Geometry: final body of the model. Coordinates: model frame, mm. A direction names the side the tool comes from. Coordinates: 2 decimals unless noted, no trailing zeros. Write each loop counter-clockwise with the first axis right and the second up, starting at its lowest first coordinate (ties: lowest second). Pieces come first, ordered by that corner, then holes.
from build123d import *

# Parameters (mm, degrees)
SKETCH1_R                = 5
BOSS_EXTRUDE1_DEPTH      = 5
BOSS_EXTRUDE2_DEPTH      = 5
BOSS_EXTRUDE2_DEPTH_BACK = 15
SKETCH2_R                = 5


with BuildPart() as part:
    # Sketch1 → Boss-Extrude1 (new, symmetric)
    with BuildSketch(Plane(origin=(0, 0, 0), x_dir=(1, 0, 0), z_dir=(0, 1, 0))):
        with BuildLine():
            Line((-216.890839392, 48.397972972), (1.736481777, 9.84807753))
            Line((1.736481777, 9.84807753), (288, 10))
            ThreePointArc((288, 10), (298, 0), (288, -10))
            Line((288, -10), (0, -10))
            ThreePointArc((0, -10), (-0.871557427, -9.961946981), (-1.736481777, -9.84807753))
            Line((-1.736481777, -9.84807753), (-220.363802945, 28.701817912))
            ThreePointArc((-220.363802945, 28.701817912), (-228.475398699, 40.286377219), (-216.890839392, 48.397972972))
        make_face()
        with Locations(Location((-218.627321169, 38.549895442, 0), (0, 0, 270))):
            Circle(SKETCH1_R, mode=Mode.SUBTRACT)
        with Locations(Location((0, 0, 0), (0, 0, 270))):
            Circle(SKETCH1_R, mode=Mode.SUBTRACT)
        with Locations(Location((288, 0, 0), (0, 0, 270))):
            Circle(SKETCH1_R, mode=Mode.SUBTRACT)
    extrude(amount=BOSS_EXTRUDE1_DEPTH, both=True)

    # Sketch2 → Boss-Extrude2 (add, two sides: drawn at the far end of the back side and taken through both)
    with BuildSketch(Plane(origin=(0, 0, 0), x_dir=(1, 0, 0), z_dir=(0, 1, 0)).offset(-BOSS_EXTRUDE2_DEPTH_BACK)):
        with Locations(Location((-218.627321169, 38.549895442, 0), (0, 0, 270))):
            Circle(SKETCH2_R)
    extrude(amount=BOSS_EXTRUDE2_DEPTH + BOSS_EXTRUDE2_DEPTH_BACK)


solid = part.part
Item 1: Pin query (flat end, axial travel): pin 1 (11.5 mm diameter, centred on x = 0, z = 0, fed in from -Y); pin 2 (6 mm diameter, centred on x = 76, y = -2.5, fed in from -Z); pin 3 (1.5 mm diameter, centred on y = -6.5, z = -16.5, fed in from +X). Return the tip coordinate at first contact, or that it passes through.
Derived:
pin 1: stops at y = -5
pin 2: stops at z = -9.89
pin 3: passes through
Item 2: Section C-C, the plane x = 95. Output: boundary loops of the cut face in (y, z), plus the area to 3 significant figures.
Derived:
outline: (-5, -9.9) - (5, -9.9) - (5, 10) - (-5, 10) - close
area: 199 mm2
Item 3: Section D-D, the plane z = -19. Output: boundary loops of the cut face in (x, y), plus the area to 3 significant figures.
Derived:
outline: (-165.34, -5) - (-50.17, -5) - (-50.17, 5) - (-165.34, 5) - close
area: 1,150 mm2
Item 4: Material intervals for probe 1 along Z at (x, y) = (288, -0.5); probe 2 along Y at (x, z) = (-44, 1); probe 3 along Z at (x, y) = (76, -3.5), sorted ascending.
Derived:
probe 1: z = -10 to -5, 5 to 10
probe 2: y = -5 to 5
probe 3: z = -9.89 to 10
Item 5: Section B-B, the plane z = 0. Output: boundary loops of the cut face in (x, y), plus the area to 3 significant figures.
Derived:
outline: (-57.59, -5) - (-5, -5) - (-5, 5) - (-57.59, 5) - close; (5, -5) - (283, -5) - (283, 5) - (5, 5) - close; (293, -5) - (298, -5) - (298, 5) - (293, 5) - close
area: 3,360 mm2
Item 6: Section A-A, the plane y = 2. Output: boundary loops of the cut face in (x, z), plus the area to 3 significant figures.
Derived:
outline: (-220.36, -28.7) arc R10 ccw to (-216.89, -48.4) - (1.74, -9.85) - (288, -10) arc R10 ccw to (288, 10) - (0, 10) arc R10 ccw to (-1.74, 9.85) - close; hole circle Ø10 at (0, 0); hole circle Ø10 at (288, 0)
area: 10,300 mm2
Item 7: Set-up query: faces 1 (the flat face through (-109.108, 0.07, -29.393)), 2 (the cylindrical face through (-213.67, -10.07, -39.2)). Return all of +Z, -Z, +X, -X, +Y, -Y with unobstructed straight access to the full face (end or side cutting, diameter ignored); none if empty.
Derived:
face 1: -Z, +X, +Y, -Y
face 2: -Y
Item 8: Pull-direction query (X, two-part tool) for faces 3 (the cylindrical face through (-4.88, -0.07, -1.08)), 4 (the flat face through (36, 5, -9)), 5 (the flat face through (-109.52, 0.07, -9.157)), 6 (the cylindrical face through (292.957, -0.07, -0.651)); classes: released by +X, released by -X, zero draft, split by the parting line, or undercut.
Derived:
face 3: undercut
face 4: zero draft
face 5: released by -X
face 6: undercut
